from build123d import *

# Parameters (mm, degrees)
BOSS_EXTRUDE1_DEPTH = 170
SKETCH3_R           = 7.5
BOSS_EXTRUDE2_DEPTH = 10
SKETCH4_R           = 7.75
CUT_EXTRUDE1_DEPTH  = 17


with BuildPart() as part:
    # Sketch1 → Boss-Extrude1 (new body)
    with BuildSketch(Plane(origin=(0, 0, 0), x_dir=(0, 0, -1), z_dir=(1, 0, 0))):
        with BuildLine():
            Line((-25, 16.583123952), (-25, -16.583123952))
            ThreePointArc((-25, -16.583123952), (0, -30), (25, -16.583123952))
            Line((25, -16.583123952), (25, 16.583123952))
            ThreePointArc((25, 16.583123952), (0, 30), (-25, 16.583123952))
        make_face()
    extrude(amount=BOSS_EXTRUDE1_DEPTH)

    # Sketch3 → Boss-Extrude2 (add)
    with BuildSketch(Plane.XY.offset(25)):
        with Locations(Location((20, 0, 0), (0, 0, 180))):
            Circle(SKETCH3_R)
    boss_extrude2 = extrude(amount=BOSS_EXTRUDE2_DEPTH)

    # Mirror1: Boss-Extrude2 across plane
    add(boss_extrude2.mirror(Plane.XY))

    # Sketch4 → Cut-Extrude1 (cut)
    with BuildSketch(Plane(origin=(170, 0, 0), x_dir=(0, 0, -1), z_dir=(1, 0, 0))):
        Circle(SKETCH4_R)
    extrude(amount=-CUT_EXTRUDE1_DEPTH, mode=Mode.SUBTRACT)


solid = part.part
Read the model definition and answer for the solid it produces. Units are mm, in the model's axes. A direction names the side the tool comes from. Round coordinates to 2 decimals unless told otherwise and drop trailing zeros. Order: outer loops, then holes, each group sorted by start corner. A loop starts at its lowest first (then second) coordinate and runs counter-clockwise, first axis right, second up. Notation, with made-up numbers: (33.5, 85.5) - (77.5, 85.5) arc R23 cw to (77.5, 99.5) - close; hole circle Ø5 at (80.5, -20). An arc over 180 degrees is marked (long way). Use one line per item in the form item = value. Start each with the question number.
(1) For faces 4 (the face through (170, -6.2, -5.2)), 5 (the face through (27.493, -0.33, -29.93)), 6 (the face through (27.493, -0.33, 29.93)), 7 (the face through (153, 0, 0)), determine the directions among +Z, -Z, +X, -X, +Y, -Y from which every point of the face is accessible in a straight line to the end or side of a thin tool.
(2) Flat-ended cylindrical pins translate along their axes: pin 1 Ø10 at (x, y) = (50, -4.5) entering from +Z; pin 2 Ø1 at (x, z) = (85, -22.5) entering from +Y; pin 3 Ø12 at (x, z) = (37.5, 18) entering from +Y. Find the tip coordinate at first contact, or state that the pin passes through.
(3) Determine the mould class of faces 1 (the face through (161.619, 7.684, 1.009)), 2 (the face through (84, 0, -25)), 3 (the face through (84, -30, 0)) for opening direction Y: +Y half, -Y half, draft (parallel to the pull), parting line (faces both ways), or undercut.
(4) The part is cut by section D-D (x = 75.5). Give the vertices of the cut face in (y, z).
(5) The part is cut by section A-A (z = 0). Give the vertices of the cut face in (x, y).
(6) The part is cut by section B-B (y = 0). Give the vertices of the cut face in (x, z).
(7) Find the intervals of material crossed by line 1 along Z through (x, y) = (131, 8.5); line 2 along Z through (x, y) = (23, -22.5); line 3 along Y through (x, z) = (138.5, 7), in increasing order. Write a range as from..to.
(8) The part is cut by section C-C (x = 20). Give the vertices of the cut face in (y, z), then the cut area to 3 significant figures.
Checked values:
q1.face_4 = +Z, -Z, +X, +Y, -Y
q1.face_5 = -Z
q1.face_6 = +Z
q1.face_7 = +X
q2.pin_1 = 25
q2.pin_2 = 20.4
q2.pin_3 = 27.5
q3.face_1 = undercut
q3.face_2 = draft
q3.face_3 = -Y half
q4.outline = (-16.58, -25) - (16.58, -25) arc R30 ccw to (16.58, 25) - (-16.58, 25) arc R30 ccw to start
q5.outline = (0, -30) - (170, -30) - (170, -7.75) - (153, -7.75) - (153, 7.75) - (170, 7.75) - (170, 30) - (0, 30) - close
q6.outline = (0, -25) - (12.5, -25) - (12.5, -35) - (27.5, -35) - (27.5, -25) - (170, -25) - (170, -7.75) - (153, -7.75) - (153, 7.75) - (170, 7.75) - (170, 25) - (27.5, 25) - (27.5, 35) - (12.5, 35) - (12.5, 25) - (0, 25) - close
q7.line_1 = -25..25
q7.line_2 = -19.84..19.84
q7.line_3 = -29.17..29.17
q8.outline = (-16.58, -25) - (-7.5, -25) - (-7.5, -35) - (7.5, -35) - (7.5, -25) - (16.58, -25) arc R30 ccw to (16.58, 25) - (7.5, 25) - (7.5, 35) - (-7.5, 35) - (-7.5, 25) - (-16.58, 25) arc R30 ccw to start
q8.area = 2,900 mm^2
